```python
from build123d import *

# Parameters (mm, degrees)
HEAD_SKETCH_R                  = 2.25
HEAD_DEPTH                     = 2
THREADED_SECTION_STUB_SKETCH_R = 1.5
THREADED_SECTION_DEPTH         = 8
END_OF_BOLT_CHAMFER_SIZE       = 0.5
END_OF_BOLT_CHAMFER_SIZE2      = 0.288675135
COSMETIC_FILLETS_R             = 0.2


with BuildPart() as part:
    # Head Sketch → Head (new body)
    with BuildSketch(Plane(origin=(0, 0, 0), x_dir=(1, 0, 0), z_dir=(0, 1, 0))):
        with Locations(Location((0, 0, 0), (0, 0, 270))):
            Circle(HEAD_SKETCH_R)
        Polygon((-0.577350269, 1), (-1.154700538, 0), (-0.577350269, -1), (0.577350269, -1), (1.154700538, 0), (0.577350269, 1), align=None, mode=Mode.SUBTRACT)
    extrude(amount=HEAD_DEPTH)

    # Threaded Section Stub Sketch → Threaded Section (add)
    with BuildSketch(Plane(origin=(0, 0, 0), x_dir=(1, 0, 0), z_dir=(0, 1, 0))):
        with Locations(Location((0, 0, 0), (0, 0, 270))):
            Circle(THREADED_SECTION_STUB_SKETCH_R)
    extrude(amount=-THREADED_SECTION_DEPTH)

    # End Of Bolt chamfer
    end_of_bolt_chamfer_edges = [part.edges().sort_by_distance(p)[0] for p in [
        (0, -8, -1.5),
    ]]
    end_of_bolt_chamfer_side = [part.faces().sort_by_distance(p)[0] for p in [
        (0, -8, 0),
    ]]
    chamfer(end_of_bolt_chamfer_edges, length=END_OF_BOLT_CHAMFER_SIZE, length2=END_OF_BOLT_CHAMFER_SIZE2, reference=end_of_bolt_chamfer_side[0])

    # Cosmetic Fillets
    cosmetic_fillets_edges = [part.edges().sort_by_distance(p)[0] for p in [
        (-0.577350269, 1, -1),
        (-0.8660254037844384, 0, 0.5000000000000003),
        (-1.154700538, 1, 0),
        (0, 0, 1),
        (-0.577350269, 1, 1),
        (0.8660254037844388, 0, 0.4999999999999998),
        (0.577350269, 1, 1),
        (0.8660254037844388, 0, -0.5000000000000002),
        (0, 2, -1),
        (-0.866025404, 2, -0.5),
        (-0.866025404, 2, 0.5),
        (0, 2, 1),
        (0.866025404, 2, 0.5),
        (0.866025404, 2, -0.5),
        (0, 0, -2.25),
        (0, 2, -2.25),
        (0, 0, -1),
        (0.577350269, 1, -1),
        (-0.8660254037844386, 0, -0.4999999999999998),
    ]]
    fillet(cosmetic_fillets_edges, radius=COSMETIC_FILLETS_R)


solid = part.part
```
Can you work these out from the model? Positions are in its coordinate system, mm. A direction names the side the tool comes from. Coordinates: 2 decimals unless noted, no trailing zeros. Order: outer loops, then holes, each group sorted by start corner. A loop starts at its lowest first (then second) coordinate and runs counter-clockwise, first axis right, second up.
1. Thinking about a two-plate mould opening in X: for faces 1 (the face through (0.676, 0.989, 2.146)), 2 (the face through (0, -8, 0)), 3 (the face through (0.9, 0.99, -0.44)), which applies, +X half, -X half, draft (parallel to the pull), parting line (faces both ways), or undercut?
2. I'm going to push flat-ended pins straight in: pin 1 (1 mm diameter, centred on y = -2, z = 1.5, fed in from -X); pin 2 (1 mm diameter, centred on x = 1.5, y = -3, fed in from -Z); pin 3 (2 mm diameter, centred on y = -6, z = 0, fed in from -X). Where does each tip first touch, or does it pass through?
3. For faces 4 (the face through (0.45, -3.8, 1.43)), 5 (the face through (0.89, 0.99, 0.46)), 6 (the face through (-1, 2, 1)), which set-ups out of +Z, -Z, +X, -X, +Y, -Y let a thin tool reach every point of the face, with its end or its side?
4. If we section it at B-B (y = -0.25): Please give me the cut outline in (x, z).
5. I need wall thicknesses on line 1 (Y direction, x = 1.3, z = 1.45); line 2 (Z direction, x = 0.15, y = 1) (3 decimals); line 3 (Z direction, x = 1, y = 1.5). Which ranges of each line are inside material? Lowest first, please.
6. If we section it at A-A (x = 0): Please give me the cut outline in (y, z).
Entries:
1. face 1: parting line
1. face 2: draft
1. face 3: undercut
2. pin 1: stops at x = -1.12
2. pin 2: stops at z = -1.12
2. pin 3: stops at x = -1.5
3. face 4: -Y
3. face 5: +Y
3. face 6: +Z, -Z, +X, -X, +Y
4. outline: circle Ø3 at (0, 0)
5. line 1: y = 0 to 2
5. line 2: z = -2.245 to -1, 1 to 2.245
5. line 3: z = -2.02 to -0.27, 0.27 to 2.02
6. outline: (-8, -1) - (-7.71, -1.5) - (0, -1.5) - (0, -2.05) arc R0.2 ccw to (0.2, -2.25) - (1.8, -2.25) arc R0.2 ccw to (2, -2.05) - (2, -1.2) arc R0.2 ccw to (1.8, -1) - (0.2, -1) arc R0.2 cw to (0, -0.8) - (0, 0.8) arc R0.2 cw to (0.2, 1) - (1.8, 1) arc R0.2 ccw to (2, 1.2) - (2, 2.05) arc R0.2 ccw to (1.8, 2.25) - (0.2, 2.25) arc R0.2 ccw to (0, 2.05) - (0, 1.5) - (-7.71, 1.5) - (-8, 1) - close
